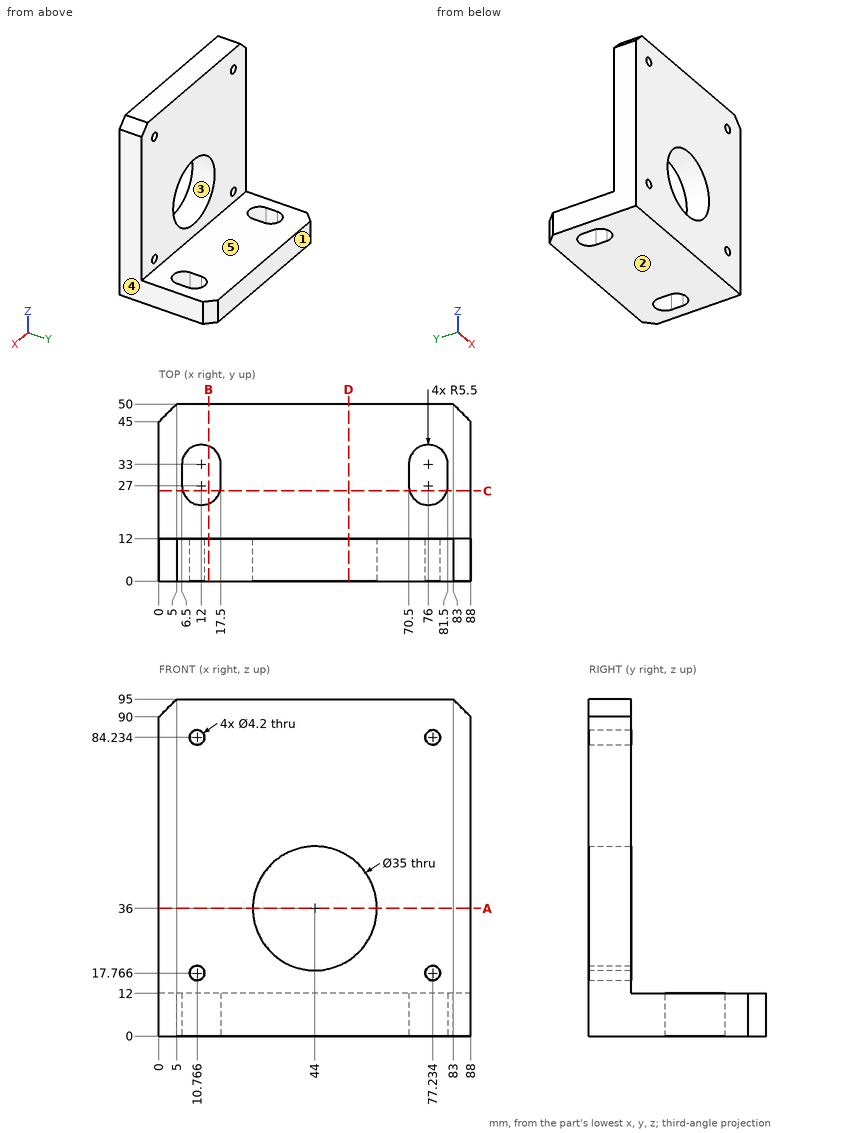
Could you check a few things on this drawing? It's one solid part, dimensions in mm from its lowest x, y, z. A direction names the side the tool comes from. Give positions to 0.01 mm unless a question says otherwise; leave off trailing zeros. Write each loop counter-clockwise with the first axis right and the second up, starting at its lowest first coordinate (ties: lowest second). Pieces come first, ordered by that corner, then holes. Notation, with made-up numbers: (81.25, 31.5) -> (125.25, 31.5) arc R33 ccw to (125.25, 61.5) -> close; hole circle Ø1 at (79.5, 62.5). An arc over 180 degrees is marked (long way). Answer as CSV lines item,"result". Start each with the question number.
(1) If we section it at D-D, the plane x = 53.5: Write out the boundary of the cut face in (y, z), and give its area (3 significant figures).
(2) I'm going to push flat-ended pins straight in: pin 1 Ø2 at (x, z) = (73.5, 66) entering from +Y; pin 2 Ø4 at (x, y) = (64, 25.5) entering from -Z; pin 3 Ø4 at (x, z) = (77.23, 84.23) entering from -Y; pin 4 Ø10 at (x, y) = (76, 34) entering from +Z. Where does each tip first touch, or does it pass through?
(3) Which directions (+Z, -Z, +X, -X, +Y, -Y) give clear straight access to the entire face, cutting with the end or side of a thin tool? Please do the marked faces 4 and 5.
(4) If we mould it in two halves opening along Z, with no side actions, what happens to the marked faces 1, 2 and 3? For each: +Z half, -Z half, draft (parallel to the pull), parting line (faces both ways), or undercut.
(5) If we section it at B-B, the plane x = 14: Write out the boundary of the cut face in (y, z).
(6) Please list where these lines run through material, in increasing order: line 1 (Y direction, x = 79, z = 75); line 2 (X direction, y = 26, z = 10).
(7) If we section it at C-C, the plane y = 25.5: Write out the boundary of the cut face in (x, z), and give its area (3 significant figures).
(8) If we section it at A-A, the plane z = 36: Write out the boundary of the cut face in (x, y), and give its area (3 significant figures).
Answer list:
1,outline,"(0, 0) -> (50, 0) -> (50, 12) -> (12, 12) -> (12, 21.3) -> (0, 21.3) -> close; (0, 50.7) -> (12, 50.7) -> (12, 95) -> (0, 95) -> close"
1,area,"1,240 mm^2"
2,pin 1,"y = 12"
2,pin 2,"z = 0"
2,pin 3,"through"
2,pin 4,"z = 12"
3,face 4,"+Z, -Z, +X, +Y, -Y"
3,face 5,"+Z, +X, -X, +Y"
4,face 1,"draft"
4,face 2,"-Z half"
4,face 3,"undercut"
5,outline,"(0, 0) -> (21.88, 0) -> (21.88, 12) -> (12, 12) -> (12, 95) -> (0, 95) -> close; (38.12, 0) -> (50, 0) -> (50, 12) -> (38.12, 12) -> close"
6,line 1,"0 to 12"
6,line 2,"0 to 6.59, 17.41 to 70.59, 81.41 to 88"
7,outline,"(0, 0) -> (6.71, 0) -> (6.71, 12) -> (0, 12) -> close; (17.29, 0) -> (70.71, 0) -> (70.71, 12) -> (17.29, 12) -> close; (81.29, 0) -> (88, 0) -> (88, 12) -> (81.29, 12) -> close"
7,area,"802 mm^2"
8,outline,"(0, 0) -> (26.5, 0) -> (26.5, 12) -> (0, 12) -> close; (61.5, 0) -> (88, 0) -> (88, 12) -> (61.5, 12) -> close"
8,area,"636 mm^2"
